from build123d import *

# Parameters (mm, degrees)
AUFSATZ_LINEAR_AUSTRAGEN1_DEPTH = 0.6
VERRUNDUNG1_R                   = 1
VERRUNDUNG2_R                   = 1


with BuildPart() as part:
    # glider-sketch → Aufsatz-Linear austragen1 (new body, symmetric)
    with BuildSketch(Plane.XY):
        Polygon((-2.5, 2.5), (-2, 2.5), (-2, 12.5), (2, 12.5), (2, 2.5), (2.5, 2.5), (2.5, -2.5), (-2.5, -2.5), align=None)
    extrude(amount=AUFSATZ_LINEAR_AUSTRAGEN1_DEPTH, both=True)

    # Verrundung1
    verrundung1_edges = [part.edges().sort_by_distance(p)[0] for p in [
        (2, 12.5, 0),
    ]]
    fillet(verrundung1_edges, radius=VERRUNDUNG1_R)

    # Verrundung2
    verrundung2_edges = [part.edges().sort_by_distance(p)[0] for p in [
        (-2, 12.5, 0),
    ]]
    fillet(verrundung2_edges, radius=VERRUNDUNG2_R)


solid = part.part
Input: part model. Units: mm. Frame: model coordinates. A direction names the side the tool comes from. Give positions to 0.01 mm unless a question says otherwise; leave off trailing zeros. Write each loop counter-clockwise with the first axis right and the second up, starting at its lowest first coordinate (ties: lowest second). Pieces come first, ordered by that corner, then holes. Notation, with made-up numbers: M 18.25,50 L 40.25,50 A25 ccw 40.25,75 Z; hole C 22.5,61.25 d6. An arc over 180 degrees is marked long. Use one line per item in the form item = value.
1. Cut plane B-B on y = 8. Return loops of the section in (x, z).
Outcome:
outline = M -2,-0.6 L 2,-0.6 L 2,0.6 L -2,0.6 Z
2. First-contact query: P1, Ø0.6, axis at y = 6.5, z = 0, coming from the -X side; P2, Ø0.6, axis at x = 2, z = 0, coming from the +Y side. Flat tips, straight axial feed; report the tip coordinate or a pass-through.
Outcome:
P1 = -2
P2 = 12.21
3. Cut plane A-A on z = -0.25. Return loops of the section in (x, y).
Outcome:
outline = M -2.5,-2.5 L 2.5,-2.5 L 2.5,2.5 L 2,2.5 L 2,11.5 A1 ccw 1,12.5 L -1,12.5 A1 ccw -2,11.5 L -2,2.5 L -2.5,2.5 Z
4. Reachability of faces 1 (the face through (0, -2.5, 0)), 2 (the face through (-2, 7, 0)), 3 (the face through (2, 7, 0)) from +Z, -Z, +X, -X, +Y, -Y: full face, straight path, thin tool, end or side. Return the list, or none.
Outcome:
face_1 = +Z, -Z, +X, -X, -Y
face_2 = +Z, -Z, -X, +Y
face_3 = +Z, -Z, +X, +Y
5. Ray query, L1, parallel to X at y = 8.5, z = -0.5; L2, parallel to Y at x = 2.15, z = 0; L3, parallel to Y at x = -1.1, z = 0. Return the intervals inside material, ascending.
Outcome:
L1 = -2 to 2
L2 = -2.5 to 2.5
L3 = -2.5 to 12.49
